from build123d import *

# Parameters (mm, degrees)
F0_R     = 2
F1_DEPTH = 3


with BuildPart() as f1:
    # F0 (on Front) → F1 (new body)
    with BuildSketch(Plane.XZ):
        with BuildLine():
            Line((-121, -93), (121, -93))
            ThreePointArc((121, -93), (130.899495, -88.899495), (135, -79))
            Line((135, -79), (135, 79))
            ThreePointArc((135, 79), (130.899495, 88.899495), (121, 93))
            Line((121, 93), (-121, 93))
            ThreePointArc((-121, 93), (-130.899495, 88.899495), (-135, 79))
            Line((-135, 79), (-135, -79))
            ThreePointArc((-135, -79), (-130.899495, -88.899495), (-121, -93))
        make_face()
        with Locations((-121, -79)):
            Circle(F0_R, mode=Mode.SUBTRACT)
        with Locations((121, -79)):
            Circle(F0_R, mode=Mode.SUBTRACT)
        with Locations((-121, 79)):
            Circle(F0_R, mode=Mode.SUBTRACT)
        Polygon((108.5, 68), (108.5, -68), (-108.5, -68), (-108.5, 68), (0, 68), align=None, mode=Mode.SUBTRACT)
        with BuildLine():
            ThreePointArc((3.5, 80.342077), (2.474874, 77.867203), (0, 76.842077))
            ThreePointArc((0, 76.842077), (-2.474874, 82.81695), (3.5, 80.342077))
        make_face(mode=Mode.SUBTRACT)
        with Locations((121, 79)):
            Circle(F0_R, mode=Mode.SUBTRACT)
    extrude(amount=F1_DEPTH)


solid = f1.part
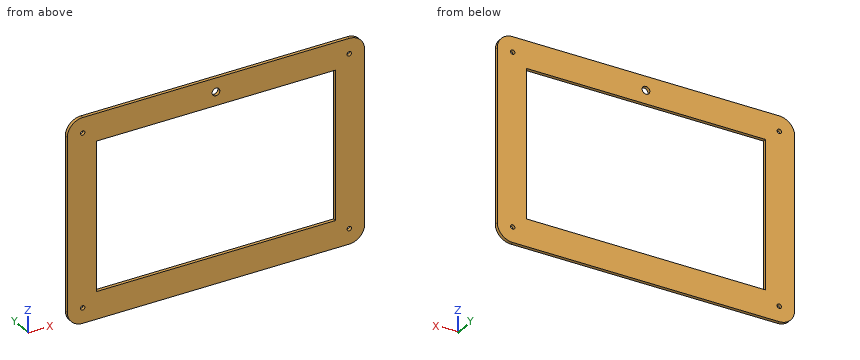
Geometry check sheet. Reference: the model listing, model coordinates, mm. Give positions to 0.01 mm unless a question says otherwise; leave off trailing zeros. Order: outer loops, then holes, each group sorted by start corner. A loop starts at its lowest first (then second) coordinate and runs counter-clockwise, first axis right, second up. Notation, with made-up numbers: M 13.5,-10 L 38.5,-10 A20 cw 38.5,4 Z; hole C 33.25,86.5 d8. An arc over 180 degrees is marked long. Use a Markdown table: item, result.
Item 1: Section check B-B (y = -0.6). Record the cut outline in (x, z), and give its area (3 significant figures).
Answers follow:
| item | result |
|---|---|
| outline | M -135,-79 A14 ccw -121,-93 L 121,-93 A14 ccw 135,-79 L 135,79 A14 ccw 121,93 L -121,93 A14 ccw -135,79 Z; hole C -121,-79 d4; hole C -121,79 d4; hole M -108.5,-68 L 108.5,-68 L 108.5,68 L -108.5,68 Z; hole C 0,80.34 d7; hole C 121,-79 d4; hole C 121,79 d4 |
| area | 20,500 mm2 |
Item 2: Section check A-A (x = 69.5). Record the cut outline in (y, z), and give its area (3 significant figures).
Answers follow:
| item | result |
|---|---|
| outline | M -3,-93 L 0,-93 L 0,-68 L -3,-68 Z; M -3,68 L 0,68 L 0,93 L -3,93 Z |
| area | 150 mm2 |
Item 3: Depth check by flat-ended pin: P1, Ø3, axis at x = 121, z = 79, coming from the +Y side. Enter the tip coordinate at first touch or a pass-through.
Answers follow:
| item | result |
|---|---|
| P1 | passes through |
Item 4: Section check C-C (z = -46). Record the cut outline in (x, y).
Answers follow:
| item | result |
|---|---|
| outline | M -135,-3 L -108.5,-3 L -108.5,0 L -135,0 Z; M 108.5,-3 L 135,-3 L 135,0 L 108.5,0 Z |
Item 5: Material ranges on line 1 along Z through (x, y) = (-121, -2.1); line 2 along Z through (x, y) = (0, -2); line 3 along Z through (x, y) = (107.5, -0.65), recorded low to high.
Answers follow:
| item | result |
|---|---|
| line 1 | z = -93 to -81, -77 to 77, 81 to 93 |
| line 2 | z = -93 to -68, 68 to 76.84, 83.84 to 93 |
| line 3 | z = -93 to -68, 68 to 93 |
